from build123d import *

# Parameters (mm, degrees)
SKETCH2_W               = 76.675
SKETCH2_H               = 86.2
SKETCH2_W_2             = 66.675
SKETCH2_H_2             = 76.2
BOSS_EXTRUDE1_DEPTH     = 152.4
CUT_EXTRUDE1_REACH      = 88.2
FILLET1_R               = 6.35
SKETCH5_R               = 2.13995
CUT_EXTRUDE2_DEPTH      = 6
LPATTERN1_COUNT         = 4
LPATTERN1_PITCH         = 38.1
MIRROR3_COPY_1_SKETCH_R = 2.13995
MIRROR3_COPY_1_DEPTH    = 6
MIRROR3_COPY_2_SKETCH_R = 2.13995
MIRROR3_COPY_2_DEPTH    = 6
MIRROR3_COPY_3_SKETCH_R = 2.13995
MIRROR3_COPY_3_DEPTH    = 6
CUT_EXTRUDE3_DEPTH      = 34.925
FILLET2_R               = 0.79375


with BuildPart() as part:
    # Sketch2 → Boss-Extrude1 (new body)
    with BuildSketch(Plane.XY):
        Rectangle(SKETCH2_W, SKETCH2_H)
        Rectangle(SKETCH2_W_2, SKETCH2_H_2, mode=Mode.SUBTRACT)
    extrude(amount=BOSS_EXTRUDE1_DEPTH)

    # Sketch3 → Cut-Extrude1 (cut, up to next)
    with BuildSketch(Plane.XZ.offset(43.1), mode=Mode.PRIVATE) as cut_extrude1_sk1:
        with BuildLine():
            Line((20, 152.4), (20, 70.8))
            ThreePointArc((20, 70.8), (0, 50.8), (-20, 70.8))
            Line((-20, 70.8), (-20, 152.4))
            ThreePointArc((-20, 152.4), (0, 172.4), (20, 152.4))
        make_face()
    cut_extrude1_tool1 = extrude(cut_extrude1_sk1.sketch, amount=-CUT_EXTRUDE1_REACH, mode=Mode.PRIVATE) & part.part
    add(cut_extrude1_tool1.solids().sort_by_distance((0, -43.1, 111.6))[0], mode=Mode.SUBTRACT)

    # Fillet1
    fillet1_edges = [part.edges().sort_by_distance(p)[0] for p in [
        (33.3375, -38.1, 76.2),
        (33.3375, 38.1, 76.2),
        (-33.3375, 38.1, 76.2),
        (-33.3375, -38.1, 76.2),
        (20, -40.6, 152.4),
        (-20, -40.6, 152.4),
        (38.3375, -43.1, 76.2),
        (-38.3375, -43.1, 76.2),
        (-38.3375, 43.1, 76.2),
        (38.3375, 43.1, 76.2),
    ]]
    fillet(fillet1_edges, radius=FILLET1_R)

    # Sketch5 → Cut-Extrude2 (cut, through all)
    with BuildSketch(Plane.XZ.offset(-38.1)):
        with Locations((-17.4625, 142.875)):
            Circle(SKETCH5_R)
    cut_extrude2 = extrude(amount=-CUT_EXTRUDE2_DEPTH, mode=Mode.SUBTRACT)

    # Sketch6 → Cut-Revolve1 (revolve, cut)
    with BuildSketch(Plane(origin=(-17.4625, 0, 0), x_dir=(0, -1, 0), z_dir=(-1, 0, 0))):
        Polygon((-38.1, 138.7475), (-38.1, 142.875), (-42.2275, 142.875), align=None)
    cut_revolve1 = revolve(axis=Axis((-17.4625, 38.1, 142.875), (0, 1, 0)), mode=Mode.SUBTRACT)

    # LPattern1: Cut-Extrude2, Cut-Revolve1 ×4
    with Locations(*[(0, 0, -i * LPATTERN1_PITCH) for i in range(1, LPATTERN1_COUNT)]):
        add(cut_extrude2, mode=Mode.SUBTRACT)
        add(cut_revolve1, mode=Mode.SUBTRACT)

    # Mirror3: Cut-Revolve1, Cut-Extrude2 across plane
    add(cut_revolve1.mirror(Plane(origin=(0, 0, 0), x_dir=(0, 0, 1), z_dir=(1, 0, 0))), mode=Mode.SUBTRACT)
    add(cut_extrude2.mirror(Plane(origin=(0, 0, 0), x_dir=(0, 0, 1), z_dir=(1, 0, 0))), mode=Mode.SUBTRACT)

    # Mirror3 copy 1 sketch → Mirror3 copy 1 (cut, through all)
    with BuildSketch(Plane(origin=(0, 38.1, -38.1), x_dir=(-1, 0, 0), z_dir=(0, -1, 0))):
        with Locations((-17.4625, -142.875)):
            Circle(MIRROR3_COPY_1_SKETCH_R)
    extrude(amount=-MIRROR3_COPY_1_DEPTH, mode=Mode.SUBTRACT)

    # Mirror3 copy 2 sketch → Mirror3 copy 2 (cut, through all)
    with BuildSketch(Plane(origin=(0, 38.1, -76.2), x_dir=(-1, 0, 0), z_dir=(0, -1, 0))):
        with Locations((-17.4625, -142.875)):
            Circle(MIRROR3_COPY_2_SKETCH_R)
    extrude(amount=-MIRROR3_COPY_2_DEPTH, mode=Mode.SUBTRACT)

    # Mirror3 copy 3 sketch → Mirror3 copy 3 (cut, through all)
    with BuildSketch(Plane(origin=(0, 38.1, -114.3), x_dir=(-1, 0, 0), z_dir=(0, -1, 0))):
        with Locations((-17.4625, -142.875)):
            Circle(MIRROR3_COPY_3_SKETCH_R)
    extrude(amount=-MIRROR3_COPY_3_DEPTH, mode=Mode.SUBTRACT)

    # Mirror3 copy 4 sketch → Mirror3 copy 4 (revolve, cut)
    with BuildSketch(Plane(origin=(17.4625, 0, -38.1), x_dir=(0, -1, 0), z_dir=(1, 0, 0))):
        Polygon((-38.1, -138.7475), (-38.1, -142.875), (-42.2275, -142.875), align=None)
    revolve(axis=Axis((17.4625, 38.1, 104.775), (0, -1, 0)), mode=Mode.SUBTRACT)

    # Mirror3 copy 5 sketch → Mirror3 copy 5 (revolve, cut)
    with BuildSketch(Plane(origin=(17.4625, 0, -76.2), x_dir=(0, -1, 0), z_dir=(1, 0, 0))):
        Polygon((-38.1, -138.7475), (-38.1, -142.875), (-42.2275, -142.875), align=None)
    revolve(axis=Axis((17.4625, 38.1, 66.675), (0, -1, 0)), mode=Mode.SUBTRACT)

    # Mirror3 copy 6 sketch → Mirror3 copy 6 (revolve, cut)
    with BuildSketch(Plane(origin=(17.4625, 0, -114.3), x_dir=(0, -1, 0), z_dir=(1, 0, 0))):
        Polygon((-38.1, -138.7475), (-38.1, -142.875), (-42.2275, -142.875), align=None)
    revolve(axis=Axis((17.4625, 38.1, 28.575), (0, -1, 0)), mode=Mode.SUBTRACT)

    # Sketch7 → Cut-Extrude3 (cut)
    with BuildSketch(Plane(origin=(0, 0, 0), x_dir=(-1, 0, 0), z_dir=(0, 0, -1))):
        with BuildLine():
            Line((38.3375, -36.75), (38.3375, 36.75))
            ThreePointArc((38.3375, 36.75), (36.477628061, 41.240128061), (31.9875, 43.1))
            Line((31.9875, 43.1), (-31.9875, 43.1))
            ThreePointArc((-31.9875, 43.1), (-36.477628061, 41.240128061), (-38.3375, 36.75))
            Line((-38.3375, 36.75), (-38.3375, -36.75))
            ThreePointArc((-38.3375, -36.75), (-36.477628061, -41.240128061), (-31.9875, -43.1))
            Line((-31.9875, -43.1), (31.9875, -43.1))
            ThreePointArc((31.9875, -43.1), (36.477628061, -41.240128061), (38.3375, -36.75))
        make_face()
    extrude(amount=-CUT_EXTRUDE3_DEPTH, mode=Mode.SUBTRACT)

    # Fillet2
    fillet2_edges = [part.edges().sort_by_distance(p)[0] for p in [
        (0, -43.1, 50.8),
        (20, -43.1, 108.425),
        (0, -38.1, 50.8),
        (20, -38.1, 108.425),
        (-38.3375, 0, 152.4),
        (0, 43.1, 152.4),
        (-29.16875, -43.1, 152.4),
        (-26.66875, -38.1, 152.4),
        (-33.3375, 0, 152.4),
        (0, 38.1, 152.4),
        (33.3375, 0, 152.4),
        (26.66875, -38.1, 152.4),
        (29.16875, -43.1, 152.4),
        (38.3375, 0, 152.4),
        (36.477628061, 41.240128061, 152.4),
        (36.477628061, -41.240128061, 152.4),
        (-36.477628061, -41.240128061, 152.4),
        (-36.477628061, 41.240128061, 152.4),
        (-20, -43.1, 108.425),
        (-21.859871939, -43.1, 150.540128061),
        (21.859871939, -43.1, 150.540128061),
        (-20, -38.1, 108.425),
        (-21.859871939, -38.1, 150.540128061),
        (21.859871939, -38.1, 150.540128061),
        (31.477628061, 36.240128061, 152.4),
        (-31.477628061, 36.240128061, 152.4),
        (-31.477628061, -36.240128061, 152.4),
        (31.477628061, -36.240128061, 152.4),
    ]]
    fillet(fillet2_edges, radius=FILLET2_R)


solid = part.part
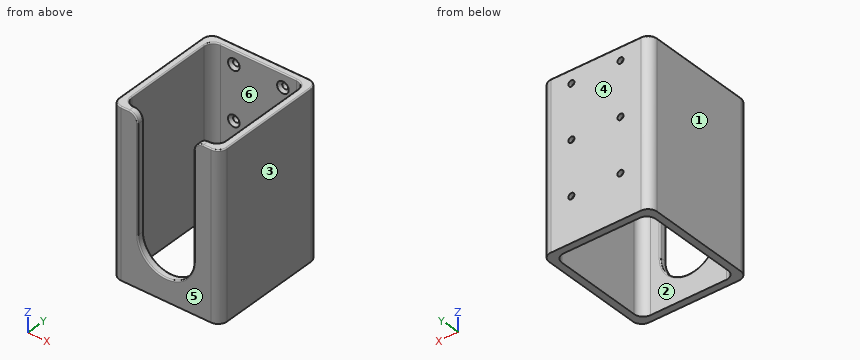
Design review of the part built by this model. Coordinates are the model's own, in mm. Face numbers are marked on the shaded views. A direction names the side the tool comes from. Give positions to 0.01 mm unless a question says otherwise; leave off trailing zeros. Order: outer loops, then holes, each group sorted by start corner. A loop starts at its lowest first (then second) coordinate and runs counter-clockwise, first axis right, second up. Notation, with made-up numbers: (60.25, 83.5) - (118.25, 83.5) arc R10 cw to (118.25, 91.5) - close; hole circle Ø8 at (-7.75, -4.5). An arc over 180 degrees is marked (long way). Write item = value, one per line. Start each with the question number.
Q1. To check wall thickness, follow L1, parallel to X at y = -3.5, z = 90; L2, parallel to Y at x = -21, z = 139; L3, parallel to Y at x = 11, z = 127. State the ranges of each line that lie inside material, in increasing order. Write a range as from..to.
Q2. Mouldability with a two-part tool opening along X and no side actions: class the marked faces 1, 2, 3 and 4 as released by +X, released by -X, zero draft, split by the parting line, or undercut.
Q3. We need section C-C on z = 98. State the section outline as (x, y) points, plus the area to 3 significant figures.
Q4. We need section A-A on x = 0. State the section outline as (y, z) points (1 decimal).
Q5. We need section B-B on y = -19. State the section outline as (x, z) points (1 decimal), plus the area to 3 significant figures.
Q6. Clearance check with flat-ended pins moving along their axes: pin 1 Ø2.5 at (x, z) = (-17.46, 142.88) entering from -Y; pin 2 Ø16 at (x, z) = (-8, 121) entering from -Y; pin 3 Ø1 at (y, z) = (-41, 112.5) entering from +X; pin 4 Ø5 at (x, z) = (-17.46, 104.78) entering from -Y. State where each tip first meets the part, or that it passes through.
Q7. Tool access review of the marked faces 5 and 6: name each direction out of +Z, -Z, +X, -X, +Y, -Y from which nothing blocks a thin tool from reaching the whole face with its end or side.
Working result:
q1.L1 = -38.34..-33.34, 33.34..38.34
q1.L2 = -43.1..-38.1, 38.1..43.1
q1.L3 = 38.1..43.1
q2.face_1 = released by -X
q2.face_2 = undercut
q2.face_3 = released by +X
q2.face_4 = zero draft
q3.outline = (-38.34, -36.75) arc R6.35 ccw to (-31.99, -43.1) - (-20.79, -43.1) arc R0.79 ccw to (-20, -42.31) - (-20, -38.89) arc R0.79 ccw to (-20.79, -38.1) - (-26.99, -38.1) arc R6.35 cw to (-33.34, -31.75) - (-33.34, 31.75) arc R6.35 cw to (-26.99, 38.1) - (26.99, 38.1) arc R6.35 cw to (33.34, 31.75) - (33.34, -31.75) arc R6.35 cw to (26.99, -38.1) - (20.79, -38.1) arc R0.79 ccw to (20, -38.89) - (20, -42.31) arc R0.79 ccw to (20.79, -43.1) - (31.99, -43.1) arc R6.35 ccw to (38.34, -36.75) - (38.34, 36.75) arc R6.35 ccw to (31.99, 43.1) - (-31.99, 43.1) arc R6.35 ccw to (-38.34, 36.75) - close
q3.area = 1,330 mm²
q4.outline = (-43.1, 34.9) - (-38.1, 34.9) - (-38.1, 50) arc R0.8 ccw to (-38.9, 50.8) - (-42.3, 50.8) arc R0.8 ccw to (-43.1, 50) - close; (38.1, 34.9) - (43.1, 34.9) - (43.1, 151.6) arc R0.8 ccw to (42.3, 152.4) - (38.9, 152.4) arc R0.8 ccw to (38.1, 151.6) - close
q5.outline = (-38.3, 34.9) - (-33.3, 34.9) - (-33.3, 151.6) arc R0.8 ccw to (-34.1, 152.4) - (-37.5, 152.4) arc R0.8 ccw to (-38.3, 151.6) - close; (33.3, 34.9) - (38.3, 34.9) - (38.3, 151.6) arc R0.8 ccw to (37.5, 152.4) - (34.1, 152.4) arc R0.8 ccw to (33.3, 151.6) - close
q5.area = 1,170 mm²
q6.pin_1 = through
q6.pin_2 = 38.1
q6.pin_3 = 37.11
q6.pin_4 = 39.72
q7.face_5 = +Z, -Z, +X, -X, -Y
q7.face_6 = +Z, -Z
